The listing builds one solid part. Answer for the finished solid, in the listing's coordinates (mm). Face numbers are marked on the shaded views. A direction names the side the tool comes from. Round coordinates to 2 decimals unless told otherwise and drop trailing zeros. Write each loop counter-clockwise with the first axis right and the second up, starting at its lowest first coordinate (ties: lowest second). Pieces come first, ordered by that corner, then holes.
from build123d import *

# Parameters (mm, degrees)
BOSS_EXTRUDE1_DEPTH          = 5
SKETCH1_3_R                  = 1.7
SKETCH1_3_R_2                = 1.25
CUT_EXTRUDE3_DEPTH           = 29.722813233
CUT_EXTRUDE4_START           = 5
SKETCH1_4_R                  = 2.6
CUT_EXTRUDE4_DEPTH           = 3.9
CUT_EXTRUDE4_DRAFT           = -1.5
CUT_EXTRUDE4_PROFILE_2_DEPTH = 3.9
CUT_EXTRUDE4_PROFILE_2_DRAFT = -1.5
CUT_EXTRUDE4_PROFILE_3_DEPTH = 3.9
CUT_EXTRUDE4_PROFILE_3_DRAFT = -1.5
CUT_EXTRUDE4_PROFILE_4_DEPTH = 3.9
CUT_EXTRUDE4_PROFILE_4_DRAFT = -1.5
FILLET1_R                    = 5
FILLET2_R                    = 1


with BuildPart() as part:
    # Sketch1 → Boss-Extrude1 (new body)
    with BuildSketch(Plane(origin=(0, -7, 0), x_dir=(-1, 0, 0), z_dir=(0, -1, 0))):
        with BuildLine():
            Line((15, 20), (-15, 20))
            ThreePointArc((-15, 20), (-18.535533906, 18.535533906), (-20, 15))
            Line((-20, 15), (-20, -15))
            ThreePointArc((-20, -15), (-18.535533906, -18.535533906), (-15, -20))
            Line((-15, -20), (15, -20))
            ThreePointArc((15, -20), (18.535533906, -18.535533906), (20, -15))
            Line((20, -15), (20, 15))
            ThreePointArc((20, 15), (18.535533906, 18.535533906), (15, 20))
        make_face()
    extrude(amount=BOSS_EXTRUDE1_DEPTH)

    # Sketch1<3> → Cut-Extrude3 (cut, through all)
    with BuildSketch(Plane(origin=(0, -7, 0), x_dir=(-1, 0, 0), z_dir=(0, -1, 0))):
        with Locations(Location((-15, 15, 0), (0, 0, 90))):
            Circle(SKETCH1_3_R)
        with Locations(Location((15, 15, 0), (0, 0, 90))):
            Circle(SKETCH1_3_R)
        with Locations(Location((-15, -15, 0), (0, 0, 90))):
            Circle(SKETCH1_3_R)
        with Locations(Location((15, -15, 0), (0, 0, 90))):
            Circle(SKETCH1_3_R)
        with Locations(Location((0, 0, 0), (0, 0, 90))):
            Circle(SKETCH1_3_R_2)
    extrude(amount=CUT_EXTRUDE3_DEPTH, mode=Mode.SUBTRACT)


with BuildPart() as cut_extrude4_tool:
    # Sketch1<4> → Cut-Extrude4 (with draft: the straight prism first)
    with BuildSketch(Plane(origin=(0, -7, 0), x_dir=(-1, 0, 0), z_dir=(0, -1, 0)).offset(CUT_EXTRUDE4_START)):
        with Locations((15, -15)):
            Circle(SKETCH1_4_R)
    extrude(amount=-CUT_EXTRUDE4_DEPTH)
    # Cut-Extrude4: the draft: its side faces are tilted about the plane it starts from
    cut_extrude4_sides = [cut_extrude4_tool.faces().sort_by_distance(p)[0] for p in [
        (-12.4, -10.05, 15),
    ]]
    draft(cut_extrude4_sides, Plane(origin=(0, -7, 0), x_dir=(-1, 0, 0), z_dir=(0, -1, 0)).offset(CUT_EXTRUDE4_START), CUT_EXTRUDE4_DRAFT)


with BuildPart() as part_1:
    add(part.part)

    # Cut-Extrude4: cut by cut_extrude4_tool
    add(cut_extrude4_tool.part, mode=Mode.SUBTRACT)


with BuildPart() as cut_extrude4_profile_2_tool:
    # Sketch1<4> → Cut-Extrude4 profile 2 (with draft: the straight prism first)
    with BuildSketch(Plane(origin=(0, -7, 0), x_dir=(-1, 0, 0), z_dir=(0, -1, 0)).offset(CUT_EXTRUDE4_START)):
        with Locations((-15, -15)):
            Circle(SKETCH1_4_R)
    extrude(amount=-CUT_EXTRUDE4_PROFILE_2_DEPTH)
    # Cut-Extrude4 profile 2: the draft: its side faces are tilted about the plane it starts from
    cut_extrude4_profile_2_sides = [cut_extrude4_profile_2_tool.faces().sort_by_distance(p)[0] for p in [
        (17.6, -10.05, 15),
    ]]
    draft(cut_extrude4_profile_2_sides, Plane(origin=(0, -7, 0), x_dir=(-1, 0, 0), z_dir=(0, -1, 0)).offset(CUT_EXTRUDE4_START), CUT_EXTRUDE4_PROFILE_2_DRAFT)


with BuildPart() as part_2:
    add(part_1.part)

    # Cut-Extrude4 profile 2: cut by cut_extrude4_profile_2_tool
    add(cut_extrude4_profile_2_tool.part, mode=Mode.SUBTRACT)


with BuildPart() as cut_extrude4_profile_3_tool:
    # Sketch1<4> → Cut-Extrude4 profile 3 (with draft: the straight prism first)
    with BuildSketch(Plane(origin=(0, -7, 0), x_dir=(-1, 0, 0), z_dir=(0, -1, 0)).offset(CUT_EXTRUDE4_START)):
        with Locations((-15, 15)):
            Circle(SKETCH1_4_R)
    extrude(amount=-CUT_EXTRUDE4_PROFILE_3_DEPTH)
    # Cut-Extrude4 profile 3: the draft: its side faces are tilted about the plane it starts from
    cut_extrude4_profile_3_sides = [cut_extrude4_profile_3_tool.faces().sort_by_distance(p)[0] for p in [
        (17.6, -10.05, -15),
    ]]
    draft(cut_extrude4_profile_3_sides, Plane(origin=(0, -7, 0), x_dir=(-1, 0, 0), z_dir=(0, -1, 0)).offset(CUT_EXTRUDE4_START), CUT_EXTRUDE4_PROFILE_3_DRAFT)


with BuildPart() as part_3:
    add(part_2.part)

    # Cut-Extrude4 profile 3: cut by cut_extrude4_profile_3_tool
    add(cut_extrude4_profile_3_tool.part, mode=Mode.SUBTRACT)


with BuildPart() as cut_extrude4_profile_4_tool:
    # Sketch1<4> → Cut-Extrude4 profile 4 (with draft: the straight prism first)
    with BuildSketch(Plane(origin=(0, -7, 0), x_dir=(-1, 0, 0), z_dir=(0, -1, 0)).offset(CUT_EXTRUDE4_START)):
        with Locations((15, 15)):
            Circle(SKETCH1_4_R)
    extrude(amount=-CUT_EXTRUDE4_PROFILE_4_DEPTH)
    # Cut-Extrude4 profile 4: the draft: its side faces are tilted about the plane it starts from
    cut_extrude4_profile_4_sides = [cut_extrude4_profile_4_tool.faces().sort_by_distance(p)[0] for p in [
        (-12.4, -10.05, -15),
    ]]
    draft(cut_extrude4_profile_4_sides, Plane(origin=(0, -7, 0), x_dir=(-1, 0, 0), z_dir=(0, -1, 0)).offset(CUT_EXTRUDE4_START), CUT_EXTRUDE4_PROFILE_4_DRAFT)


with BuildPart() as part_4:
    add(part_3.part)

    # Cut-Extrude4 profile 4: cut by cut_extrude4_profile_4_tool
    add(cut_extrude4_profile_4_tool.part, mode=Mode.SUBTRACT)

    # Fillet1
    fillet1_edges = [part_4.edges().sort_by_distance(p)[0] for p in [
        (0, -12, 1.25),
    ]]
    fillet(fillet1_edges, radius=FILLET1_R - 0.0001)  # a hair under: the kernel refuses the full size

    # Fillet2
    fillet2_edges = [part_4.edges().sort_by_distance(p)[0] for p in [
        (-18.535533906, -12, 18.535533906),
        (-20, -12, 0),
        (-18.535533906, -12, -18.535533906),
        (0, -12, -20),
        (18.535533906, -12, -18.535533906),
        (20, -12, 0),
        (18.535533906, -12, 18.535533906),
        (0, -12, 20),
    ]]
    fillet(fillet2_edges, radius=FILLET2_R)


solid = part_4.part
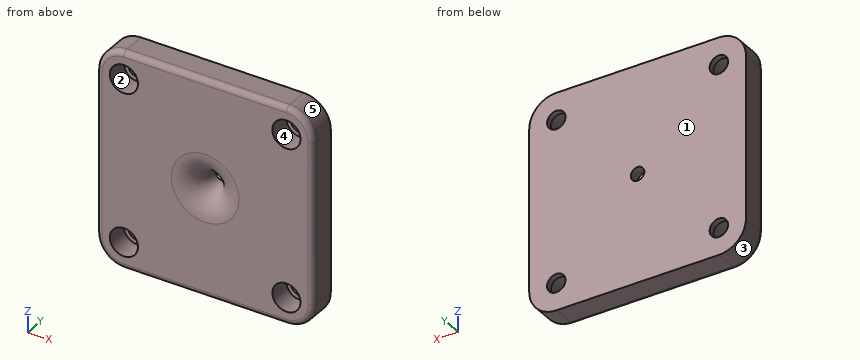
1. Section C-C on y = -8.7 is taken. Determine the outline of the cut face in (x, z).
Geometry says:
outline: (-20, -15) arc R5 ccw to (-15, -20) - (15, -20) arc R5 ccw to (20, -15) - (20, 15) arc R5 ccw to (15, 20) - (-15, 20) arc R5 ccw to (-20, 15) - close; hole circle Ø5.03 at (-15, -15); hole circle Ø5.03 at (-15, 15); hole circle Ø3.1 at (0, 0); hole circle Ø5.03 at (15, -15); hole circle Ø5.03 at (15, 15)
2. A tool of negligible diameter and unlimited length cuts with its end or side. For the marked faces 1 and 2, from which of +Z, -Z, +X, -X, +Y, -Y can it reach the whole face along a straight path? Write none if from no direction.
Geometry says:
face 1: +Z, -Z, +X, -X, +Y
face 2: -Y
3. For a pull along X with two mould halves and no side action, classify the marked faces 3, 4 and 5 as released by +X, released by -X, zero draft, split by the parting line, or undercut.
Geometry says:
face 3: released by -X
face 4: undercut
face 5: released by +X
4. Given pin 1 (5.5 mm diameter, centred on x = -16, z = -16, fed in from -Y); pin 2 (1.5 mm diameter, centred on x = 14, z = -16, fed in from -Y); pin 3 (2.5 mm diameter, centred on x = -15, z = -15, fed in from -Y), each flat-ended and moving along its own axis, determine where each tip first touches the part or whether it passes through.
Geometry says:
pin 1: stops at y = -12
pin 2: stops at y = -8.1
pin 3: passes through
5. Straight lines are drawn through the part: line 1 along X through (y, z) = (-7.5, 15); line 2 along X through (y, z) = (-8.7, 16). For each, find the intervals that lie inside material, in ascending order.
Geometry says:
line 1: x = -20 to -16.7, -13.3 to 13.3, 16.7 to 20
line 2: x = -19.9 to -17.31, -12.69 to 12.69, 17.31 to 19.9
6. Section D-D on x = -15.5 is taken. Give the number of separate pieces and of enclosed holes in the cut face, plus the area to 3 significant figures.
Geometry says:
separate pieces: 3
enclosed holes: 0
area: 153 mm2
